from build123d import *

# Parameters (mm, degrees)
F0_W     = 304.8
F0_H     = 254
F1_DEPTH = 19.05
F2_W     = 38.1
F2_H     = 127
F3_DEPTH = 19.051
F4_R     = 4.7625
F5_DEPTH = 19.051


with BuildPart() as f1:
    # F0 (on Top) → F1 (new body)
    with BuildSketch(Plane.XY):
        Rectangle(F0_W, F0_H)
    extrude(amount=F1_DEPTH)

    # F2 (on face) → F3 (cut, through all)
    with BuildSketch(Plane.XY.offset(19.05)):
        with Locations((-152.4, 0)):
            Rectangle(F2_W, F2_H)
    extrude(amount=-F3_DEPTH, mode=Mode.SUBTRACT)

    # F4 (on face) → F5 (cut, through all)
    with BuildSketch(Plane.XY.offset(19.05)):
        with Locations((19.05, 31.75)):
            Circle(F4_R)
        with Locations((19.05, -31.75)):
            Circle(F4_R)
    extrude(amount=-F5_DEPTH, mode=Mode.SUBTRACT)


solid = f1.part
The model under review builds one solid part; all positions refer to its coordinate system, in mm. A direction names the side the tool comes from. Round coordinates to 2 decimals unless told otherwise and drop trailing zeros. Write each loop counter-clockwise with the first axis right and the second up, starting at its lowest first coordinate (ties: lowest second). Pieces come first, ordered by that corner, then holes. Notation, with made-up numbers: (84.5, 45.5) -> (112.5, 45.5) arc R32 cw to (112.5, 84.5) -> close; hole circle Ø1 at (-27.5, 54.25). An arc over 180 degrees is marked (long way). Answer as a JSON object with one key per item and string values.
1. The part is to be moulded in two halves that separate along Y. For faces 3 (the face through (-143, 63.5, 10)), 4 (the face through (-2, -127, 9)), 5 (the face through (-2, 127, 9)), 6 (the face through (-152.4, -96, 9)), say which applies: pulls with the +Y half, pulls with the -Y half, needs draft (parallel to the pull), parting line crosses it, or undercut.
Results found:
{"face 3": "undercut", "face 4": "pulls with the -Y half", "face 5": "pulls with the +Y half", "face 6": "needs draft"}
2. Clearance check with flat-ended pins moving along their axes: pin 1 (5 mm diameter, centred on x = 93, y = 95.5, fed in from -Z); pin 2 (3 mm diameter, centred on y = -59.5, z = 2.5, fed in from -X). State where each tip first meets the part, or that it passes through.
Results found:
{"pin 1": "stops at z = 0", "pin 2": "stops at x = -133.35"}
3. To check wall thickness, follow line 1 along Y through (x, z) = (19.05, 15); line 2 along X through (y, z) = (63, 9.5); line 3 along X through (y, z) = (-35, 11). State the ranges of each line that lie inside material, in increasing order.
Results found:
{"line 1": "y = -127 to -36.51, -26.99 to 26.99, 36.51 to 127", "line 2": "x = -133.35 to 152.4", "line 3": "x = -133.35 to 15.57, 22.53 to 152.4"}
4. We need section A-A on y = 31.75. State the section outline as (x, z) points.
Results found:
{"outline": "(-133.35, 0) -> (14.29, 0) -> (14.29, 19.05) -> (-133.35, 19.05) -> close; (23.81, 0) -> (152.4, 0) -> (152.4, 19.05) -> (23.81, 19.05) -> close"}
5. We need section C-C on z = 4.5. State how many separate pieces and enclosed holes the cut face has, and give its area (3 significant figures).
Results found:
{"separate pieces": "1", "enclosed holes": "2", "area": "74,900 mm^2"}
6. Machinability: for faces 1 (the face through (-2, 2, 19.05)), 2 (the face through (-133.35, -1, 10)), which of the approach directions +Z, -Z, +X, -X, +Y, -Y give a long, thin tool a straight path to every point of the face, cutting with its end or side? Answer none if there is none.
Results found:
{"face 1": "+Z, +X, -X, +Y, -Y", "face 2": "+Z, -Z, -X"}
7. We need section B-B on x = 19.05. State the section outline as (y, z) points, and give its area (3 significant figures).
Results found:
{"outline": "(-127, 0) -> (-36.51, 0) -> (-36.51, 19.05) -> (-127, 19.05) -> close; (-26.99, 0) -> (26.99, 0) -> (26.99, 19.05) -> (-26.99, 19.05) -> close; (36.51, 0) -> (127, 0) -> (127, 19.05) -> (36.51, 19.05) -> close", "area": "4,480 mm^2"}
